```python
from build123d import *

# Parameters (mm, degrees)
F2_R = 4.99999


# Not quite as in the source:
# - a fillet or chamfer is up to 0.001 mm smaller than in the source, because OpenCascade refuses the exact size


with BuildPart() as f1:
    # F0 (on Front) → F1 (revolve)
    with BuildSketch(Plane.XZ):
        Polygon((-70, 25), (-90, 0), (0, 0), (0, 45), (-15, 45), (-15, 40), (-20, 40), (-20, 35), align=None)
    revolve(axis=Axis((0, 0, 22.5), (0, 0, -1)))

    # F2 (radius 5 in the source; OpenCascade refuses exactly that, so slightly less here)
    f2_edges = [f1.edges().sort_by_distance(p)[0] for p in [
        (20, 0, 40),
        (15, 0, 45),
    ]]
    fillet(f2_edges, radius=F2_R)


solid = f1.part
```
Verification items for the finished model (mm, model axes). Coordinates: 2 decimals unless noted, no trailing zeros. Loops run counter-clockwise (first coordinate to the right, second up) from the corner with the lowest first, then second, coordinate; pieces in that order, holes last. Notation, with made-up numbers: (40, 44) - (78, 44) arc R26 ccw to (78, 78) - close; hole circle Ø3 at (-38.5, -29). An arc over 180 degrees is marked (long way). Put each result on its own line as item: value.
Item 1: Gauge pin test, flat ends, axial feed: pin 1 Ø10 at (y, z) = (42, 21) entering from -X; pin 2 Ø1.5 at (x, y) = (-54, -39) entering from -Z; pin 3 Ø5 at (x, z) = (-48.5, 20) entering from -Y (3 decimals); pin 4 Ø2 at (x, z) = (-14, 12) entering from +Y. Record the tip position at first contact, or that the pin passes through.
Conclusion:
pin 1: stops at x = -65.71
pin 2: stops at z = 0
pin 3: stops at y = -59.215
pin 4: stops at y = 80
Item 2: Section check C-C (z = 9.5). Enter the section's corners in (x, y), then the cut area to 3 significant figures.
Conclusion:
outline: circle Ø164.8 at (0, 0)
area: 21,300 mm2
Item 3: Scan lines: line 1 along Z through (x, y) = (59, 37.5); line 2 along Y through (x, z) = (64, 11); line 3 along Y through (x, z) = (54.5, 23.5). Record each from-to range of solid material in increasing order.
Conclusion:
line 1: z = 0 to 25.02
line 2: y = -49.97 to 49.97
line 3: y = -45.82 to 45.82
Item 4: Section check D-D (z = 28). Enter the section's corners in (x, y).
Conclusion:
outline: circle Ø110 at (0, 0)
